from build123d import *

# Parameters (mm, degrees)
EXTRUDE_1_DEPTH     = 2
SKETCH_2_R          = 1
CUT_EXTRUDE_1_DEPTH = 2
EXTRUDE_2_DEPTH     = 7.5
SKETCH_4_R          = 1.5
SKETCH_4_R_2        = 0.25
CUT_EXTRUDE_2_DEPTH = 7.5
SKETCH_5_W          = 21
SKETCH_5_H          = 7.5
EXTRUDE_3_DEPTH     = 1.7
SKETCH_6_R          = 2
SKETCH_6_R_2        = 0.75
EXTRUDE_4_DEPTH     = 5.6
FILLET_1_R          = 2
FILLET_2_R          = 3
FILLET_3_R          = 1
FILLET_4_R          = 0.5


with BuildPart() as part:
    # 草图1 → 凸台-拉伸1 (new body)
    with BuildSketch(Plane.XY):
        Polygon((0, 10.8), (-9.8, 10.8), (-9.8, 5.8), (-12.8, 5.8), (-12.8, -5.8), (-9.8, -5.8), (-9.8, -10.8), (0, -10.8), (9.8, -10.8), (9.8, -5.8), (12.8, -5.8), (12.8, 5.8), (9.8, 5.8), (9.8, 10.8), align=None)
    extrude(amount=EXTRUDE_1_DEPTH)

    # 草图2 → 切除-拉伸1 (cut)
    with BuildSketch(Plane.XY.offset(2)):
        with Locations((-7.5, 8.3)):
            Circle(SKETCH_2_R)
        with Locations(Location((7.5, 8.3, 0), (0, 0, 180))):
            Circle(SKETCH_2_R)
        with Locations((7.5, -8.3)):
            Circle(SKETCH_2_R)
        with Locations(Location((-7.5, -8.3, 0), (0, 0, 180))):
            Circle(SKETCH_2_R)
    extrude(amount=-CUT_EXTRUDE_1_DEPTH, mode=Mode.SUBTRACT)

    # 草图3 → 凸台-拉伸2 (add)
    with BuildSketch(Plane.XY.offset(2)):
        Polygon((11.25, -3.75), (-11.25, -3.75), (-11.25, 2.25), (-9.75, 3.75), (9.75, 3.75), (11.25, 2.25), align=None)
    extrude(amount=EXTRUDE_2_DEPTH)

    # 草图4 → 切除-拉伸2 (cut)
    with BuildSketch(Plane.XY.offset(9.5)):
        with Locations((-7.5, 0)):
            Circle(SKETCH_4_R)
        with Locations((-2, 2)):
            Circle(SKETCH_4_R_2)
        with Locations(Location((2, 2, 0), (0, 0, 180))):
            Circle(SKETCH_4_R_2)
        with Locations((7.5, 0)):
            Circle(SKETCH_4_R)
        with Locations((2, -2)):
            Circle(SKETCH_4_R_2)
        with Locations(Location((-2, -2, 0), (0, 0, 180))):
            Circle(SKETCH_4_R_2)
    extrude(amount=-CUT_EXTRUDE_2_DEPTH, mode=Mode.SUBTRACT)

    # 草图5 → 凸台-拉伸3 (add)
    with BuildSketch(Plane(origin=(0, 0, 0), x_dir=(-1, 0, 0), z_dir=(0, 0, -1))):
        Rectangle(SKETCH_5_W, SKETCH_5_H)
    extrude(amount=EXTRUDE_3_DEPTH)

    # 草图6 → 凸台-拉伸4 (add)
    with BuildSketch(Plane(origin=(0, 0, -1.7), x_dir=(-1, 0, 0), z_dir=(0, 0, -1))):
        with Locations(Location((-7.5, 0, 0), (0, 0, 180))):
            Circle(SKETCH_6_R)
        with Locations(Location((-2, 2, 0), (0, 0, 180))):
            Circle(SKETCH_6_R_2)
        with Locations(Location((2, 2, 0), (0, 0, 180))):
            Circle(SKETCH_6_R_2)
        with Locations(Location((7.5, 0, 0), (0, 0, 180))):
            Circle(SKETCH_6_R)
        with Locations(Location((2, -2, 0), (0, 0, 180))):
            Circle(SKETCH_6_R_2)
        with Locations(Location((-2, -2, 0), (0, 0, 180))):
            Circle(SKETCH_6_R_2)
    extrude(amount=EXTRUDE_4_DEPTH)

    # 圆角1
    fillet_1_edges = [part.edges().sort_by_distance(p)[0] for p in [
        (9.8, 10.8, 1),
        (9.8, -10.8, 1),
        (-9.8, -10.8, 1),
        (-9.8, 10.8, 1),
    ]]
    fillet(fillet_1_edges, radius=FILLET_1_R)

    # 圆角2
    fillet_2_edges = [part.edges().sort_by_distance(p)[0] for p in [
        (-9.8, -5.8, 1),
        (9.8, -5.8, 1),
        (-9.8, 5.8, 1),
        (9.8, 5.8, 1),
    ]]
    fillet(fillet_2_edges, radius=FILLET_2_R - 0.0001)  # a hair under: the kernel refuses the full size

    # 圆角3
    fillet_3_edges = [part.edges().sort_by_distance(p)[0] for p in [
        (-10.5, -3.75, -0.85),
        (-10.5, 3.75, -0.85),
        (10.5, 3.75, -0.85),
        (10.5, -3.75, -0.85),
    ]]
    fillet(fillet_3_edges, radius=FILLET_3_R)

    # 圆角4
    fillet_4_edges = [part.edges().sort_by_distance(p)[0] for p in [
        (12.8, 5.8, 1),
        (12.8, -5.8, 1),
        (-12.8, -5.8, 1),
        (-12.8, 5.8, 1),
        (11.25, 2.25, 5.75),
        (9.75, 3.75, 5.75),
        (-9.75, 3.75, 5.75),
        (-11.25, 2.25, 5.75),
        (-11.25, -3.75, 5.75),
        (11.25, -3.75, 5.75),
    ]]
    fillet(fillet_4_edges, radius=FILLET_4_R)


solid = part.part
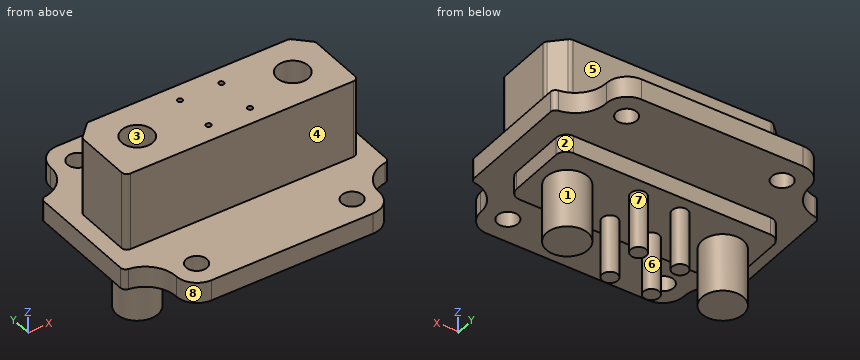
The model under review builds one solid part; all positions refer to its coordinate system, in mm. Face numbers are marked on the shaded views. A direction names the side the tool comes from. Round coordinates to 2 decimals unless told otherwise and drop trailing zeros. Loops run counter-clockwise (first coordinate to the right, second up) from the corner with the lowest first, then second, coordinate; pieces in that order, holes last. Notation, with made-up numbers: M 56.5,42 L 70.5,42 A31 ccw 70.5,70 Z; hole C -29,75 d9. An arc over 180 degrees is marked long. Answer as CSV lines item,"result". Start each with the question number.
Item 1: Consider section D-D (y = -8.3). Write out the cut boundary in (x, z).
Item 2: Consider section B-B (y = 0). Write out the cut boundary in (x, z).
Item 3: Insertion check: P1, Ø1.5, axis at x = -1, z = 4, coming from the -Y side; P2, Ø1.9, axis at x = -0.5, z = -1, coming from the +Y side; P3, Ø3, axis at x = -7.5, y = 8.3, coming from the -Z side; P4, Ø1.8, axis at x = 7.5, y = 8.3, coming from the -Z side. Each pin has a flat end and moves straight along its axis. Give the tip position at first contact, or say it passes through.
Item 4: For the marked faces 1, 2, 3 and 4, list the 3-axis set-ups (+Z, -Z, +X, -X, +Y, -Y) from which the entire face can be reached by the end or side of a thin tool; tool diameter is ignored.
Item 5: Wall thickness on line 1 (Y direction, x = 2, z = 7.5); line 2 (Z direction, x = 2.75, y = -6.75); line 3 (Z direction, x = -6.75, y = 3): over which ranges is each line inside the solid? List them lowest first. Write a range as [from, to].
Item 6: Consider section C-C (z = -2.75). Write out the cut boundary in (x, y).
Item 7: Consider section A-A (x = -7.5). Write out the cut boundary in (y, z).
Item 8: Mouldability with a two-part tool opening along X and no side actions: class the marked faces 5, 6, 7 and 8 as released by +X, released by -X, zero draft, split by the parting line, or undercut.
Answer:
1,outline,"M -9.84,0 L -8.5,0 L -8.5,2 L -9.84,2 Z; M -6.5,0 L 6.5,0 L 6.5,2 L -6.5,2 Z; M 8.5,0 L 9.84,0 L 9.84,2 L 8.5,2 Z"
2,outline,"M -12.8,0 L -10.5,0 L -10.5,-1.7 L -9.5,-1.7 L -9.5,-7.3 L -5.5,-7.3 L -5.5,-1.7 L 5.5,-1.7 L 5.5,-7.3 L 9.5,-7.3 L 9.5,-1.7 L 10.5,-1.7 L 10.5,0 L 12.8,0 L 12.8,2 L 11.25,2 L 11.25,9.5 L 9,9.5 L 9,2 L 6,2 L 6,9.5 L -6,9.5 L -6,2 L -9,2 L -9,9.5 L -11.25,9.5 L -11.25,2 L -12.8,2 Z"
3,P1,"stops at y = -3.75"
3,P2,"stops at y = 3.75"
3,P3,"stops at z = 0"
3,P4,"passes through"
4,face 1,"-Z"
4,face 2,"-Z, +X, +Y"
4,face 3,"+Z"
4,face 4,"+Z, +X, -X, -Y"
5,line 1,"y = [-3.75, -2.25], [-1.75, 1.75], [2.25, 3.75]"
5,line 2,"z = [0, 2]"
5,line 3,"z = [-1.7, 9.5]"
6,outline,"C -7.5,0 d4; C -2,-2 d1.5; C -2,2 d1.5; C 2,-2 d1.5; C 2,2 d1.5; C 7.5,0 d4"
7,outline,"M -10.8,0 L -9.3,0 L -9.3,2 L -10.8,2 Z; M -7.3,0 L -3.75,0 L -3.75,-1.7 L -2,-1.7 L -2,-7.3 L 2,-7.3 L 2,-1.7 L 3.75,-1.7 L 3.75,0 L 7.3,0 L 7.3,2 L 3.75,2 L 3.75,9.5 L 1.5,9.5 L 1.5,2 L -1.5,2 L -1.5,9.5 L -3.75,9.5 L -3.75,2 L -7.3,2 Z; M 9.3,0 L 10.8,0 L 10.8,2 L 9.3,2 Z"
8,face 5,"zero draft"
8,face 6,"undercut"
8,face 7,"undercut"
8,face 8,"released by -X"
